Can you work these out from the model? Positions are in its coordinate system, mm. Coordinates: 2 decimals unless noted, no trailing zeros. Loops run counter-clockwise (first coordinate to the right, second up) from the corner with the lowest first, then second, coordinate; pieces in that order, holes last.
```python
from build123d import *

# Parameters (mm, degrees)
SKETCH2_W           = 15
SKETCH2_H           = 3.597222937
BOSS_EXTRUDE1_DEPTH = 26.4
CUT_EXTRUDE1_DEPTH  = 26.4


with BuildPart() as part:
    # Sketch2 → Boss-Extrude1 (new body)
    with BuildSketch(Plane.XY):
        with Locations((50.434775134, 23.107461061)):
            Rectangle(SKETCH2_W, SKETCH2_H)
    extrude(amount=-BOSS_EXTRUDE1_DEPTH)

    # Sketch3 → Cut-Extrude1 (cut)
    with BuildSketch(Plane.XY):
        with BuildLine():
            Line((44.266306929, 21.308849592), (56.603243339, 21.308849592))
            ThreePointArc((56.603243339, 21.308849592), (50.434775134, 24.106072529), (44.266306929, 21.308849592))
        make_face()
    extrude(amount=-CUT_EXTRUDE1_DEPTH, mode=Mode.SUBTRACT)


solid = part.part
```
Item 1: Suppose I cut it at D-D, the plane y = 23.75. Please give me the cut outline in (x, z).
Results are:
outline: (42.93, -26.4) - (48.04, -26.4) - (48.04, 0) - (42.93, 0) - close; (52.82, -26.4) - (57.93, -26.4) - (57.93, 0) - (52.82, 0) - close
Item 2: We'd pull the mould along X, two halves only. Please class faces 1 (the face through (57.935, 23, -13)), 2 (the face through (42.935, 23, -13)), 3 (the face through (50.533, 24.105, -13.015)), 4 (the face through (57, 21.309, -13)): +X half, -X half, draft (parallel to the pull), parting line (faces both ways), or undercut.
Results are:
face 1: +X half
face 2: -X half
face 3: undercut
face 4: draft
Item 3: Suppose I cut it at C-C, the plane x = 51.5. Please give me the cut outline in (y, z), plus the area to 3 significant figures.
Results are:
outline: (24.04, -26.4) - (24.91, -26.4) - (24.91, 0) - (24.04, 0) - close
area: 23.0 mm2
Item 4: I'm going to push flat-ended pins straight in: P1, Ø6, axis at x = 49, z = -6, coming from the -Y side; P2, Ø1, axis at x = 44.5, z = -11.5, coming from the -Y side. Where does each tip first touch, or does it pass through?
Results are:
P1: stops at y = 22.8
P2: stops at y = 21.31
Item 5: Suppose I cut it at A-A, the plane y = 21.65. Please give me the cut outline in (x, z), plus the area to 3 significant figures.
Results are:
outline: (42.93, -26.4) - (44.58, -26.4) - (44.58, 0) - (42.93, 0) - close; (56.29, -26.4) - (57.93, -26.4) - (57.93, 0) - (56.29, 0) - close
area: 87.0 mm2
Item 6: Suppose I cut it at B-B, the plane z = -10. Please give me the cut outline in (x, y), plus the area to 3 significant figures.
Results are:
outline: (42.93, 21.31) - (44.27, 21.31) arc R8.2 cw to (56.6, 21.31) - (57.93, 21.31) - (57.93, 24.91) - (42.93, 24.91) - close
area: 30.0 mm2
Item 7: I need wall thicknesses on line 1 along X through (y, z) = (22.2, -4); line 2 along X through (y, z) = (22.7, -15); line 3 along Y through (x, z) = (50.5, -11.5). Which ranges of each line are inside material? Lowest first, please.
Results are:
line 1: x = 42.93 to 45.18, 55.69 to 57.93
line 2: x = 42.93 to 45.84, 55.03 to 57.93
line 3: y = 24.11 to 24.91
